Geometry check sheet. Reference: drawing and pictorial views, mm from the part's lowest x, y, z. Coordinates: 2 decimals unless noted, no trailing zeros. Write each loop counter-clockwise with the first axis right and the second up, starting at its lowest first coordinate (ties: lowest second). Pieces come first, ordered by that corner, then holes. Notation, with made-up numbers: (62.5, 80) -> (98.5, 80) arc R36 cw to (98.5, 118) -> close; hole circle Ø1 at (88.25, 33.25). An arc over 180 degrees is marked (long way). Answer in a Markdown table with one row per item.
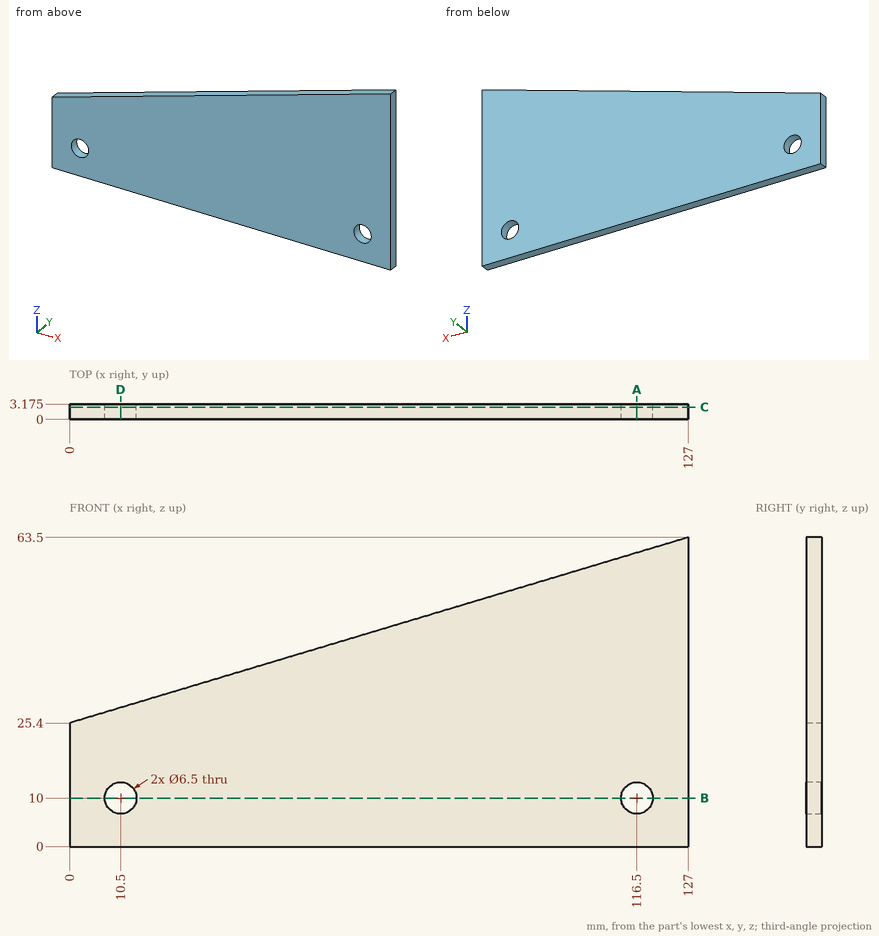
1. Section check D-D, the plane x = 10.5. Record the boundary of the cut face in (y, z) (3 decimals), plus the area to 3 significant figures.
Geometry says:
| item | result |
|---|---|
| outline | (0, 0) -> (3.175, 0) -> (3.175, 6.75) -> (0, 6.75) -> close; (0, 13.25) -> (3.175, 13.25) -> (3.175, 28.55) -> (0, 28.55) -> close |
| area | 70.0 mm^2 |
2. Section check C-C, the plane y = 2.55. Record the boundary of the cut face in (x, z), plus the area to 3 significant figures.
Geometry says:
| item | result |
|---|---|
| outline | (0, 0) -> (127, 0) -> (127, 63.5) -> (0, 25.4) -> close; hole circle Ø6.5 at (10.5, 10); hole circle Ø6.5 at (116.5, 10) |
| area | 5,580 mm^2 |
3. Thickness scan on line 1 (X direction, y = 1.9, z = 10); line 2 (X direction, y = 2.9, z = 12.5); line 3 (Z direction, x = 9.5, y = 2.15). Record the ranges inside material, lowest first. Write a range as from..to.
Geometry says:
| item | result |
|---|---|
| line 1 | 0..7.25, 13.75..113.25, 119.75..127 |
| line 2 | 0..8.42, 12.58..114.42, 118.58..127 |
| line 3 | 0..6.91, 13.09..28.25 |
4. Section check B-B, the plane z = 10. Record the boundary of the cut face in (x, y) (3 decimals), plus the area to 3 significant figures.
Geometry says:
| item | result |
|---|---|
| outline | (0, 0) -> (7.25, 0) -> (7.25, 3.175) -> (0, 3.175) -> close; (13.75, 0) -> (113.25, 0) -> (113.25, 3.175) -> (13.75, 3.175) -> close; (119.75, 0) -> (127, 0) -> (127, 3.175) -> (119.75, 3.175) -> close |
| area | 362 mm^2 |
5. Depth check by flat-ended pin: P1, Ø6, axis at x = 10.5, z = 10, coming from the -Y side. Enter the tip coordinate at first touch or a pass-through.
Geometry says:
| item | result |
|---|---|
| P1 | through |
6. Section check A-A, the plane x = 116.5. Record the boundary of the cut face in (y, z) (3 decimals).
Geometry says:
| item | result |
|---|---|
| outline | (0, 0) -> (3.175, 0) -> (3.175, 6.75) -> (0, 6.75) -> close; (0, 13.25) -> (3.175, 13.25) -> (3.175, 60.35) -> (0, 60.35) -> close |
